from build123d import *

# Parameters (mm, degrees)
BOSS_EXTRUDE1_DEPTH    = 3.175
M2_5_CLEARANCE_HOLE1_D = 2.7
M2_CLEARANCE_HOLE1_D   = 2.2


with BuildPart() as part:
    # Sketch1 → Boss-Extrude1 (new body)
    with BuildSketch(Plane.XY):
        Polygon((0, 0), (0, 9.25), (-41, 9.25), (-41, 22), (3.175, 22), (3.175, 0), align=None)
    extrude(amount=BOSS_EXTRUDE1_DEPTH)

    # M2.5 Clearance Hole1 (through all)
    with Locations(Plane.XY.offset(3.175)):
        with Locations((-38, 15.25), (-26, 15.25)):
            Hole(M2_5_CLEARANCE_HOLE1_D / 2)

    # M2 Clearance Hole1 (through all)
    with Locations(Plane.XY.offset(3.175)):
        with Locations((1.5875, 17), (1.5875, 5)):
            Hole(M2_CLEARANCE_HOLE1_D / 2)


solid = part.part
Part model, mm, in its own coordinate system. Give positions to 0.01 mm unless a question says otherwise; leave off trailing zeros. Order: outer loops, then holes, each group sorted by start corner. A loop starts at its lowest first (then second) coordinate and runs counter-clockwise, first axis right, second up. Notation, with made-up numbers: (-35.5, 42.5) - (-24.5, 42.5) arc R13 ccw to (-24.5, 55.5) - close; hole circle Ø6 at (60, 31.25). An arc over 180 degrees is marked (long way). One line per question, with ' | ' between items.
1. Band-saw the part on C-C on z = 2.25. Give the number of separate pieces and of enclosed holes in the cut face, then the cut area to 3 significant figures.
Filled in:
separate pieces: 1 | enclosed holes: 4 | area: 574 mm²
2. Band-saw the part on D-D on y = 5. List the corners of the cut face in (x, z) (1 decimal).
Filled in:
outline: (0, 0) - (0.5, 0) - (0.5, 3.2) - (0, 3.2) - close; (2.7, 0) - (3.2, 0) - (3.2, 3.2) - (2.7, 3.2) - close
3. Drill centre lines: probe 1 along Y at (x, z) = (-26, 2.05); probe 2 along Y at (x, z) = (-20.5, 0.2); probe 3 along X at (y, z) = (15.75, 1.75) (3 decimals). Where is each one in solid material? Low to high.
Filled in:
probe 1: 9.25 to 13.9, 16.6 to 22 | probe 2: 9.25 to 22 | probe 3: -41 to -39.254, -36.746 to -27.254, -24.746 to 3.175
4. Pull direction Y, two halves, no side cores. Call faces 1 (the face through (-20, 9.25, 2)), 2 (the face through (-37.824, 16.589, 1.565)), 3 (the face through (0, 5, 2)): +Y half, -Y half, draft (parallel to the pull), parting line (faces both ways), or undercut.
Filled in:
face 1: -Y half | face 2: undercut | face 3: draft
5. Band-saw the part on A-A on y = 15.25. List the corners of the cut face in (x, z) (3 decimals).
Filled in:
outline: (-41, 0) - (-39.35, 0) - (-39.35, 3.175) - (-41, 3.175) - close; (-36.65, 0) - (-27.35, 0) - (-27.35, 3.175) - (-36.65, 3.175) - close; (-24.65, 0) - (3.175, 0) - (3.175, 3.175) - (-24.65, 3.175) - close
6. Band-saw the part on B-B on x = -26. List the corners of the cut face in (y, z) (3 decimals), then the cut area to 3 significant figures.
Filled in:
outline: (9.25, 0) - (13.9, 0) - (13.9, 3.175) - (9.25, 3.175) - close; (16.6, 0) - (22, 0) - (22, 3.175) - (16.6, 3.175) - close | area: 31.9 mm²
